For this review, take the finished solid that the model builds, in its own axes (mm). A direction names the side the tool comes from. Give positions to 0.01 mm unless a question says otherwise; leave off trailing zeros. Loops run counter-clockwise (first coordinate to the right, second up) from the corner with the lowest first, then second, coordinate; pieces in that order, holes last.
```python
from build123d import *

# Parameters (mm, degrees)
SKETCH1_W           = 107.95
SKETCH1_H           = 25.4
BOSS_EXTRUDE1_DEPTH = 9.525
SKETCH3_W           = 107.95
SKETCH3_H           = 6.35
CUT_EXTRUDE2_DEPTH  = 10.525
SKETCH5_R           = 1.524
CUT_EXTRUDE4_DEPTH  = 10.525
SKETCH6_W           = 107.95
SKETCH6_H           = 6.35
BOSS_EXTRUDE2_DEPTH = 9.525
SKETCH7_W           = 9.525
SKETCH7_H           = 9.525
SKETCH7_R           = 1.524
BOSS_EXTRUDE3_DEPTH = 9.525
SKETCH8_R           = 2.0955
CUT_EXTRUDE5_DEPTH  = 10.525
FILLET3_R           = 0.254


with BuildPart() as part:
    # Sketch1 → Boss-Extrude1 (new body)
    with BuildSketch(Plane(origin=(0, 0, 0), x_dir=(1, 0, 0), z_dir=(0, 1, 0))):
        Rectangle(SKETCH1_W, SKETCH1_H)
    extrude(amount=BOSS_EXTRUDE1_DEPTH)

    # Sketch3 → Cut-Extrude2 (cut, through all)
    with BuildSketch(Plane.XZ):
        with Locations((0, 9.525)):
            Rectangle(SKETCH3_W, SKETCH3_H)
    extrude(amount=-CUT_EXTRUDE2_DEPTH, mode=Mode.SUBTRACT)

    # Sketch5 → Cut-Extrude4 (cut, through all)
    with BuildSketch(Plane(origin=(0, 9.525, 0), x_dir=(1, 0, 0), z_dir=(0, 1, 0))):
        with Locations((44.45, 3.175)):
            Circle(SKETCH5_R)
        with Locations((-44.45, 3.175)):
            Circle(SKETCH5_R)
    extrude(amount=-CUT_EXTRUDE4_DEPTH, mode=Mode.SUBTRACT)

    # Sketch6 → Boss-Extrude2 (add, through all)
    with BuildSketch(Plane(origin=(0, 9.525, 0), x_dir=(1, 0, 0), z_dir=(0, 1, 0))):
        with Locations((0, 15.875)):
            Rectangle(SKETCH6_W, SKETCH6_H)
        with Locations((0, -9.525)):
            Rectangle(SKETCH6_W, SKETCH6_H)
    extrude(amount=-BOSS_EXTRUDE2_DEPTH)

    # Sketch7 → Boss-Extrude3 (add, through all)
    with BuildSketch(Plane(origin=(0, 9.525, 0), x_dir=(1, 0, 0), z_dir=(0, 1, 0))):
        with Locations((58.7375, 14.2875)):
            Rectangle(SKETCH7_W, SKETCH7_H)
        with Locations((58.7375, 14.2875)):
            Circle(SKETCH7_R, mode=Mode.SUBTRACT)
        with Locations((58.7375, -7.9375)):
            Rectangle(SKETCH7_W, SKETCH7_H)
        with Locations((58.7375, -7.9375)):
            Circle(SKETCH7_R, mode=Mode.SUBTRACT)
        with Locations((-58.7375, -7.9375)):
            Rectangle(SKETCH7_W, SKETCH7_H)
        with Locations((-58.7375, -7.9375)):
            Circle(SKETCH7_R, mode=Mode.SUBTRACT)
        with Locations((-58.7375, 14.2875)):
            Rectangle(SKETCH7_W, SKETCH7_H)
        with Locations((-58.7375, 14.2875)):
            Circle(SKETCH7_R, mode=Mode.SUBTRACT)
    extrude(amount=-BOSS_EXTRUDE3_DEPTH)

    # Sketch8 → Cut-Extrude5 (cut, through all)
    with BuildSketch(Plane(origin=(0, 0, 0), x_dir=(-1, 0, 0), z_dir=(0, -1, 0))):
        with Locations((55.860468878, -2.2606)):
            Circle(SKETCH8_R)
        with Locations((55.860468878, 8.6106)):
            Circle(SKETCH8_R)
    cut_extrude5 = extrude(amount=-CUT_EXTRUDE5_DEPTH, mode=Mode.SUBTRACT)

    # Mirror1: Cut-Extrude5 across plane
    add(cut_extrude5.mirror(Plane(origin=(0, 0, 0), x_dir=(0, 0, 1), z_dir=(1, 0, 0))), mode=Mode.SUBTRACT)

    # Fillet3
    fillet3_edges = [part.edges().sort_by_distance(p)[0] for p in [
        (-63.5, 4.7625, -9.525),
        (-63.5, 4.7625, -19.05),
        (-57.745937756, 4.7625, -9.525),
        (-57.745937756, 4.7625, 3.175),
        (-53.975, 4.7625, 1.3462),
        (-53.975, 4.7625, -7.6962),
        (57.745937756, 4.7625, 3.175),
        (57.745937756, 4.7625, -9.525),
        (53.975, 4.7625, 1.3462),
        (53.975, 4.7625, -7.6962),
        (63.5, 4.7625, -19.05),
        (63.5, 4.7625, -9.525),
        (63.5, 4.7625, 3.175),
        (63.5, 4.7625, 12.7),
        (-63.5, 4.7625, 12.7),
        (-63.5, 4.7625, 3.175),
    ]]
    fillet(fillet3_edges, radius=FILLET3_R)


solid = part.part
```
Item 1: Clearance check with flat-ended pins moving along their axes: pin 1 Ø2 at (y, z) = (8, -7.5) entering from +X (3 decimals); pin 2 Ø1.8 at (x, z) = (-44.45, -3.175) entering from +Y. State where each tip first meets the part, or that it passes through.
Answer:
pin 1: stops at x = 53.975
pin 2: passes through
Item 2: The part is to be moulded in two halves that separate along Z. For faces 4 (the cylindrical face through (-57.284, 4.829, -14.745)), 5 (the flat face through (-1, 9.525, -3)), 6 (the flat face through (-1, 5, -19.05)), 7 (the flat face through (-1, 5, 12.7)), say which applies: released by +Z, released by -Z, zero draft, split by the parting line, or undercut.
Answer:
face 4: undercut
face 5: zero draft
face 6: released by -Z
face 7: released by +Z
Item 3: Take a section at A-A on x = -44.45. Give the boundary of the cut face in (y, z) (3 decimals), and give its area (3 significant figures).
Answer:
outline: (0, -19.05) - (9.525, -19.05) - (9.525, -4.699) - (0, -4.699) - close; (0, -1.651) - (9.525, -1.651) - (9.525, 12.7) - (0, 12.7) - close
area: 273 mm2
Item 4: For L1, parallel to X at y = 4, z = 8; L2, parallel to X at y = 2.5, z = 8.5; L3, parallel to X at y = 7.5, z = 0.5 (3 decimals), list the stretches that pass through material, from the lowest coordinate up.
Answer:
L1: x = -63.5 to -60.26, -57.21 to 57.21, 60.26 to 63.5
L2: x = -63.5 to -60.15, -57.32 to 57.32, 60.15 to 63.5
L3: x = -53.975 to 53.975
Item 5: Take a section at C-C on y = 3.5. State how many separate pieces and enclosed holes the cut face has, and give its area (3 significant figures).
Answer:
separate pieces: 1
enclosed holes: 6
area: 3,730 mm2
Item 6: Take a section at B-B on z = -0.5. Give the boundary of the cut face in (x, y) (3 decimals).
Answer:
outline: (-53.975, 0) - (53.975, 0) - (53.975, 9.525) - (-53.975, 9.525) - close
Item 7: Tool access review of faces 1 (the flat face through (-61, 5, 3.175)), 2 (the flat face through (53.975, 5, -3)), 3 (the cylindrical face through (-54.866, 4.696, 4.105)): name each direction out of +Z, -Z, +X, -X, +Y, -Y from which nothing blocks a thin tool from reaching the whole face with its end or side.
Answer:
face 1: -X, +Y, -Y
face 2: +X, +Y, -Y
face 3: +Y, -Y
